from build123d import *

# Parameters (mm, degrees)
SKETCH1_R           = 16
BOSS_EXTRUDE3_DEPTH = 5
SKETCH4_R           = 7.5
BOSS_EXTRUDE4_DEPTH = 40
SKETCH5_R           = 1.75
CUT_EXTRUDE2_DEPTH  = 5
SKETCH6_R           = 4
CUT_EXTRUDE3_DEPTH  = 45
SKETCH7_R           = 3
CUT_EXTRUDE4_DEPTH  = 3.1
CHAMFER1_SIZE       = 0.25


with BuildPart() as part:
    # Sketch1 → Boss-Extrude3 (new body)
    with BuildSketch(Plane(origin=(0, 0, 0), x_dir=(1, 0, 0), z_dir=(0, 1, 0))):
        Circle(SKETCH1_R)
    extrude(amount=BOSS_EXTRUDE3_DEPTH)

    # Sketch4 → Boss-Extrude4 (add)
    with BuildSketch(Plane(origin=(0, 5, 0), x_dir=(1, 0, 0), z_dir=(0, 1, 0))):
        Circle(SKETCH4_R)
    extrude(amount=BOSS_EXTRUDE4_DEPTH)

    # Sketch5 → Cut-Extrude2 (cut)
    with BuildSketch(Plane(origin=(0, 5, 0), x_dir=(1, 0, 0), z_dir=(0, 1, 0))):
        with Locations((0, 12)):
            Circle(SKETCH5_R)
        with Locations((-12, 0)):
            Circle(SKETCH5_R)
        with Locations((12, 0)):
            Circle(SKETCH5_R)
        with Locations((0, -12)):
            Circle(SKETCH5_R)
    extrude(amount=-CUT_EXTRUDE2_DEPTH, mode=Mode.SUBTRACT)

    # Sketch6 → Cut-Extrude3 (cut)
    with BuildSketch(Plane(origin=(0, 45, 0), x_dir=(1, 0, 0), z_dir=(0, 1, 0))):
        Circle(SKETCH6_R)
    extrude(amount=-CUT_EXTRUDE3_DEPTH, mode=Mode.SUBTRACT)

    # Sketch7 → Cut-Extrude4 (cut)
    with BuildSketch(Plane.XZ):
        with Locations((0, 12)):
            Circle(SKETCH7_R)
        with Locations((-12, 0)):
            Circle(SKETCH7_R)
        with Locations((0, -12)):
            Circle(SKETCH7_R)
        with Locations((12, 0)):
            Circle(SKETCH7_R)
    extrude(amount=-CUT_EXTRUDE4_DEPTH, mode=Mode.SUBTRACT)

    # Chamfer1
    chamfer1_edges = [part.edges().sort_by_distance(p)[0] for p in [
        (-16, 5, 0),
        (-7.5, 45, 0),
    ]]
    chamfer(chamfer1_edges, length=CHAMFER1_SIZE)


solid = part.part
CAD build for the part. Positions are in the model's coordinates, mm. A direction names the side the tool comes from. Coordinates: 2 decimals unless noted, no trailing zeros. Write each loop counter-clockwise with the first axis right and the second up, starting at its lowest first coordinate (ties: lowest second). Pieces come first, ordered by that corner, then holes. Notation, with made-up numbers: M -38,-38.5 L -19,-38.5 A14 ccw -19,-30.5 Z; hole C 60.25,40 d8. An arc over 180 degrees is marked long. Answer as a JSON object with one key per item and string values. Group by question number.
1) Saw through at C-C (y = 28). Write the cut outline in (x, z), plus the area to 3 significant figures.
2) Tool access for faces 1 (the face through (-7.493, 24.597, -0.33)), 2 (the face through (3, 0, 3)), 3 (the face through (14, 3.1, 0)): list every direction of +Z, -Z, +X, -X, +Y, -Y with a clear straight run to the whole face (end or side of a thin tool).
3) Pin check, flat tips, straight feed: pin 1 Ø2 at (x, z) = (-10, -13) entering from -Y; pin 2 Ø7 at (x, z) = (0, 12) entering from +Y; pin 3 Ø1.8 at (x, z) = (-11.5, 1.5) entering from -Y; pin 4 Ø1.5 at (y, z) = (5, -2) entering from -X. Stop position of each tip, or through.
4) Wall check: line 1 (Z direction, x = 0, y = 1); line 2 (X direction, y = 32, z = 0); line 3 (Z direction, x = -12, y = 2.55). Give the ranges that are in metal, low to high. Write a range as from..to.
5) Saw through at A-A (z = 0). Give the number of separate pieces and of enclosed holes in the cut face, plus the area to 3 significant figures.
6) Mould opens along X. For faces 4 (the face through (7, 5, -4)), 5 (the face through (-0.228, 4.063, -13.735)), 6 (the face through (0, 3.1, -14)), 7 (the face through (-3.47, 2.34, 15.62)) say: +X half, -X half, draft (parallel to the pull), parting line (faces both ways), or undercut.
Values follow:
{
 "1": {"outline": "C 0,0 d15; hole C 0,0 d8", "area": "126 mm2"},
 "2": {"face 1": "+Y", "face 2": "+Z, -Z, +X, -X, -Y", "face 3": "-Y"},
 "3": {"pin 1": "stops at y = 0", "pin 2": "stops at y = 5", "pin 3": "stops at y = 3.1", "pin 4": "stops at x = -15.95"},
 "4": {"line 1": "z = -16..-15, -9..-4, 4..9, 15..16", "line 2": "x = -7.5..-4, 4..7.5", "line 3": "z = -10.58..-3, 3..10.58"},
 "5": {"separate pieces": "4", "enclosed holes": "0", "area": "349 mm2"},
 "6": {"face 4": "draft", "face 5": "undercut", "face 6": "undercut", "face 7": "parting line"}
}
